Here's the drawing with two shaded views (mm, measured from the low corner). I have some questions. A direction names the side the tool comes from. Round coordinates to 2 decimals unless told otherwise and drop trailing zeros. Order: outer loops, then holes, each group sorted by start corner. A loop starts at its lowest first (then second) coordinate and runs counter-clockwise, first axis right, second up.
Q1. If we section it at D-D (x = 30.5): Please give me the cut outline in (y, z) (1 decimal).
Q2. For the marked faces 1 and 2, which set-ups out of +Z, -Z, +X, -X, +Y, -Y let a thin tool reach every point of the face, with its end or its side?
Q3. We'd pull the mould along X, two halves only. Please class the marked faces 3, 4 and 5: pulls with the +X half, pulls with the -X half, needs draft (parallel to the pull), parting line crosses it, or undercut.
Q4. If we section it at B-B (y = 4.5): Count the separate pieces of the cut face and the enclosed holes in it, plus the area to 3 significant figures.
Q5. If we section it at C-C (x = 44): Please give me the cut outline in (y, z) (1 decimal).
Q6. If I drill on line 1 (Z direction, x = 50, y = 5.5); line 2 (X direction, y = 5.75, z = 61.5) (1 decimal); line 3 (Y direction, x = 77.5, z = 40.5), over which ranges is the centre line in solid material (lowest first)?
Q7. Will these pins go through, and if not, where does the flat tip stop? P1, Ø21.5, axis at x = 33, z = 46, coming from the +Y side; P2, Ø1, axis at x = 23, y = 4, coming from the +Z side; P3, Ø1, axis at x = 9.5, z = 22.5, coming from the +Y side.
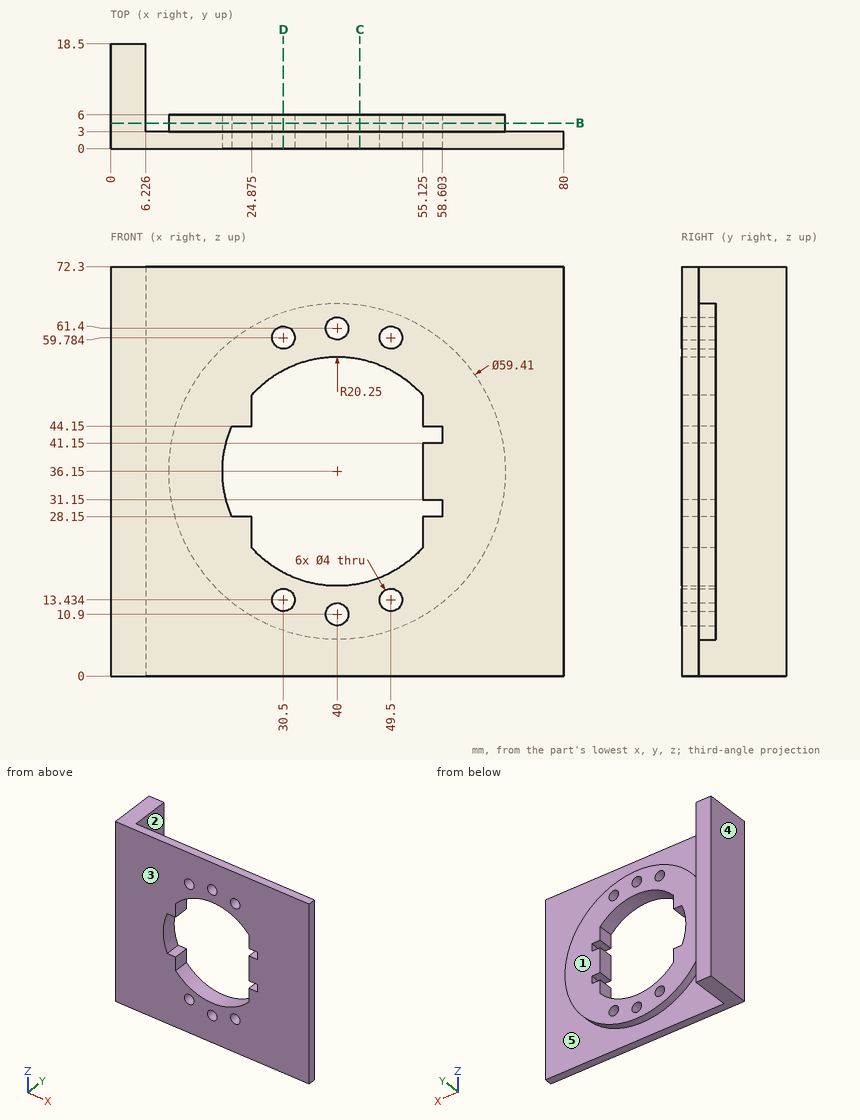
Solution:
1. outline: (0, 0) - (3, 0) - (3, 8) - (6, 8) - (6, 11.4) - (0, 11.4) - close; (0, 15.4) - (6, 15.4) - (6, 18.3) - (0, 18.3) - close; (0, 54) - (6, 54) - (6, 57.8) - (0, 57.8) - close; (0, 61.8) - (6, 61.8) - (6, 64.3) - (3, 64.3) - (3, 72.3) - (0, 72.3) - close
2. face 1: +Z, -Z, +X, +Y
2. face 2: +Z, -Z, +Y
3. face 3: needs draft
3. face 4: pulls with the -X half
3. face 5: undercut
4. separate pieces: 2
4. enclosed holes: 7
4. area: 1,950 mm2
5. outline: (0, 0) - (3, 0) - (3, 6.7) - (6, 6.7) - (6, 16.3) - (0, 16.3) - close; (0, 56) - (6, 56) - (6, 65.6) - (3, 65.6) - (3, 72.3) - (0, 72.3) - close
6. line 1: z = 8.18 to 11.5, 15.37 to 18.54, 53.76 to 57.85, 61.72 to 64.12
6. line 2: x = 0 to 6.2, 24.5 to 29.5, 31.5 to 38, 42 to 48.5, 50.5 to 55.5
6. line 3: y = 0 to 3
7. P1: stops at y = 6
7. P2: stops at z = 60.85
7. P3: stops at y = 3
